Study the drawing (mm; zero at the part's minimum x, y, z) and answer. A direction names the side the tool comes from. Round coordinates to 2 decimals unless told otherwise and drop trailing zeros. Write each loop counter-clockwise with the first axis right and the second up, starting at its lowest first coordinate (ties: lowest second). Pieces come first, ordered by that corner, then holes.
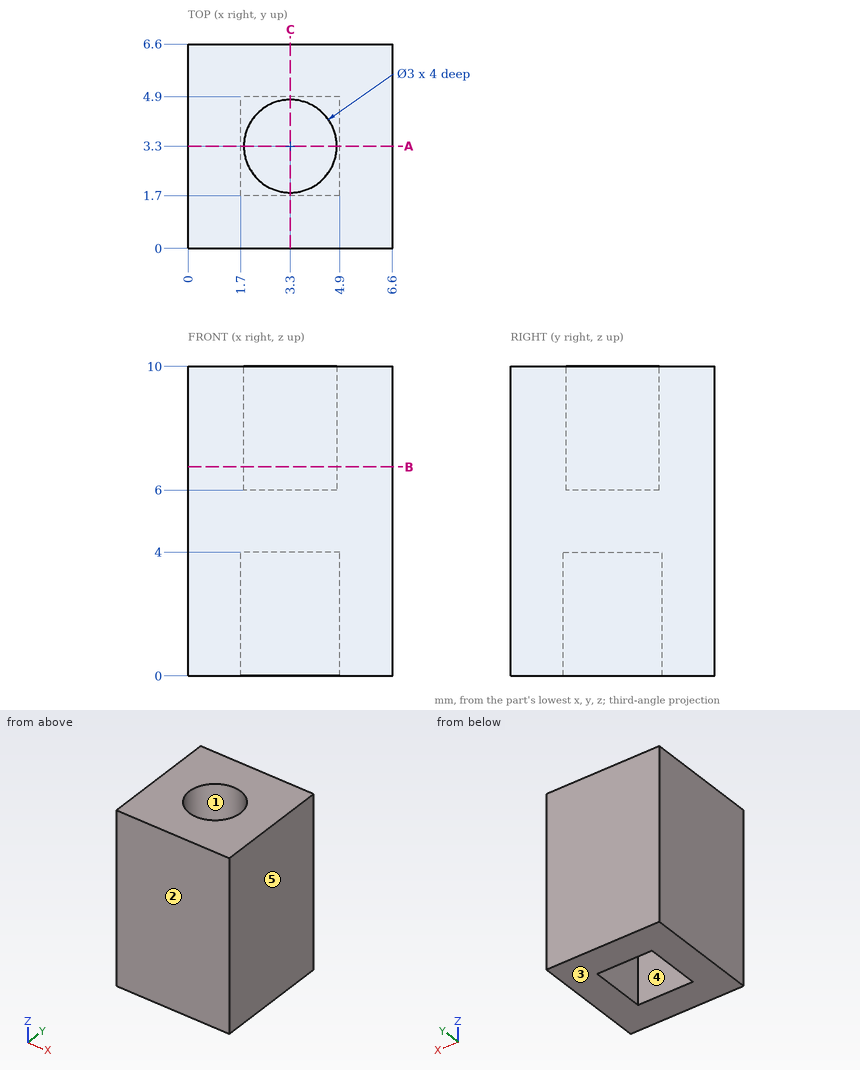
1. Section B-B on z = 6.75 is taken. Determine the outline of the cut face in (x, y).
Geometry says:
outline: (0, 0) - (6.6, 0) - (6.6, 6.6) - (0, 6.6) - close; hole circle Ø3 at (3.3, 3.3)
2. Straight lines are drawn through the part: line 1 along Y through (x, z) = (3.3, 8.6); line 2 along Z through (x, y) = (4.5, 3); line 3 along X through (y, z) = (4.25, 6.5). For each, find the intervals that lie inside material, in ascending order.
Geometry says:
line 1: y = 0 to 1.8, 4.8 to 6.6
line 2: z = 4 to 6
line 3: x = 0 to 2.14, 4.46 to 6.6
3. Section A-A on y = 3.3 is taken. Determine the outline of the cut face in (x, z), plus the area to 3 significant figures.
Geometry says:
outline: (0, 0) - (1.7, 0) - (1.7, 4) - (4.9, 4) - (4.9, 0) - (6.6, 0) - (6.6, 10) - (4.8, 10) - (4.8, 6) - (1.8, 6) - (1.8, 10) - (0, 10) - close
area: 41.2 mm2
4. A tool of negligible diameter and unlimited length cuts with its end or side. For the marked faces 4 and 5, from which of +Z, -Z, +X, -X, +Y, -Y can it reach the whole face along a straight path? Write none if from no direction.
Geometry says:
face 4: -Z
face 5: +Z, -Z, +X, +Y, -Y
5. Given pin 1 (2.5 mm diameter, centred on x = 3.3, y = 3.3, fed in from +Z), flat-ended and moving along its own axis, determine where the tip first touches the part or whether it passes through.
Geometry says:
pin 1: stops at z = 6
6. For a pull along Y with two mould halves and no side action, classify the marked faces 1, 2 and 3 as released by +Y, released by -Y, zero draft, split by the parting line, or undercut.
Geometry says:
face 1: undercut
face 2: released by -Y
face 3: zero draft
